Can you work these out from the model? Positions are in its coordinate system, mm. Face numbers are marked on the shaded views. A direction names the side the tool comes from. Round coordinates to 2 decimals unless told otherwise and drop trailing zeros. Write each loop counter-clockwise with the first axis right and the second up, starting at its lowest first coordinate (ties: lowest second). Pieces come first, ordered by that corner, then holes.
Q1. If we section it at B-B (z = 4): Please give me the cut outline in (x, y), plus the area to 3 significant figures.
Q2. We'd pull the mould along Y, two halves only. Please class the marked faces 1, 2, 3 and 4: +Y half, -Y half, draft (parallel to the pull), parting line (faces both ways), or undercut.
Q3. For the marked faces 5, 6 and 7, which set-ups out of +Z, -Z, +X, -X, +Y, -Y let a thin tool reach every point of the face, with its end or its side?
Q4. If we section it at D-D (y = 0.5): Please give me the cut outline in (x, z).
Q5. If we section it at A-A (x = -9.5): Please give me the cut outline in (y, z).
Q6. Please list where these lines run through material, in increasing order: line 1 along Y through (x, z) = (1.75, 26.75); line 2 along Z through (x, y) = (-7.5, -0.25); line 3 along Z through (x, y) = (0, 4.3).
Q7. If we section it at C-C (z = 9.5): Please give me the cut outline in (x, y).
Q8. I'm going to push flat-ended pins straight in: pin 1 Ø2.5 at (x, y) = (0, 0) entering from -Z; pin 2 Ø1.8 at (y, z) = (-0.5, 5) entering from -X; pin 3 Ø4 at (x, y) = (0, -1.5) entering from +Z. Where does each tip first touch, or does it pass through?
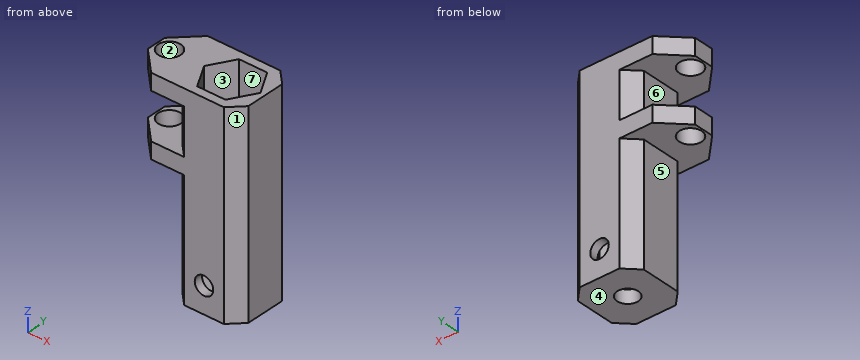
from build123d import *

# Parameters (mm, degrees)
ESQUISSE1_W             = 10
ESQUISSE1_H             = 10
BOSS_EXTRU_1_DEPTH      = 30
ENL_V_MAT_EXTRU_1_DEPTH = 28
ESQUISSE3_R             = 1.6
ENL_V_MAT_EXTRU_2_DEPTH = 31.822070015
ESQUISSE4_W             = 2.5
ESQUISSE4_H             = 10
BOSS_EXTRU_2_DEPTH      = 6.5
CHANFREIN2_SIZE         = 3.5
ESQUISSE5_R             = 1.7
ENL_V_MAT_EXTRU_3_DEPTH = 22.937410968
CHANFREIN3_SIZE         = 2
ESQUISSE9_R             = 1.4
ENL_V_MAT_EXTRU_4_DEPTH = 10


with BuildPart() as part:
    # Esquisse1 → Boss.-Extru.1 (new body)
    with BuildSketch(Plane.XY):
        Rectangle(ESQUISSE1_W, ESQUISSE1_H)
    extrude(amount=BOSS_EXTRU_1_DEPTH)

    # Esquisse2 → Enlèv. mat.-Extru.1 (cut)
    with BuildSketch(Plane.XY.offset(30)):
        Polygon((-4.272391992, 0), (-2.136195996, -3.7), (2.136195996, -3.7), (4.272391992, 0), (2.136195996, 3.7), (-2.136195996, 3.7), align=None)
    extrude(amount=-ENL_V_MAT_EXTRU_1_DEPTH, mode=Mode.SUBTRACT)

    # Esquisse3 → Enlèv. mat.-Extru.2 (cut, through all)
    with BuildSketch(Plane(origin=(0, 0, 0), x_dir=(-1, 0, 0), z_dir=(0, 0, -1))):
        Circle(ESQUISSE3_R)
    extrude(amount=-ENL_V_MAT_EXTRU_2_DEPTH, mode=Mode.SUBTRACT)

    # Esquisse4 → Boss.-Extru.2 (add)
    with BuildSketch(Plane.ZY.offset(5)):
        with Locations((28.75, 0)):
            Rectangle(ESQUISSE4_W, ESQUISSE4_H)
        with Locations((19.25, 0)):
            Rectangle(ESQUISSE4_W, ESQUISSE4_H)
    extrude(amount=BOSS_EXTRU_2_DEPTH)

    # Chanfrein2
    chanfrein2_edges = [part.edges().sort_by_distance(p)[0] for p in [
        (-11.5, -5, 28.75),
        (-11.5, 5, 28.75),
        (-11.5, -5, 19.25),
        (-11.5, 5, 19.25),
    ]]
    chamfer(chanfrein2_edges, length=CHANFREIN2_SIZE)

    # Esquisse5 → Enlèv. mat.-Extru.3 (cut, through all)
    with BuildSketch(Plane(origin=(0, 0, 18), x_dir=(-1, 0, 0), z_dir=(0, 0, -1))):
        with Locations(Location((9.5, 0, 0), (0, 0, 90))):
            Circle(ESQUISSE5_R)
    extrude(amount=-ENL_V_MAT_EXTRU_3_DEPTH, mode=Mode.SUBTRACT)

    # Chanfrein3
    chanfrein3_edges = [part.edges().sort_by_distance(p)[0] for p in [
        (-5, 5, 24),
        (-5, -5, 24),
        (5, -5, 15),
        (5, 5, 15),
        (-5, 5, 9),
        (-5, -5, 9),
    ]]
    chamfer(chanfrein3_edges, length=CHANFREIN3_SIZE)

    # Esquisse9 → Enlèv. mat.-Extru.4 (cut)
    with BuildSketch(Plane(origin=(0, 5, 0), x_dir=(1, 0, 0), z_dir=(0, 1, 0))):
        with Locations(Location((0, -4, 0), (0, 0, 180))):
            Circle(ESQUISSE9_R)
    extrude(amount=-ENL_V_MAT_EXTRU_4_DEPTH, mode=Mode.SUBTRACT)


solid = part.part
A:
1. outline: (-5, -3) - (-3, -5) - (-1.4, -5) - (-1.4, -3.7) - (-2.14, -3.7) - (-4.27, 0) - (-2.14, 3.7) - (-1.4, 3.7) - (-1.4, 5) - (-3, 5) - (-5, 3) - close; (1.4, -5) - (3, -5) - (5, -3) - (5, 3) - (3, 5) - (1.4, 5) - (1.4, 3.7) - (2.14, 3.7) - (4.27, 0) - (2.14, -3.7) - (1.4, -3.7) - close
1. area: 37.3 mm2
2. face 1: -Y half
2. face 2: undercut
2. face 3: undercut
2. face 4: draft
3. face 5: -Z, -X, +Y, -Y
3. face 6: -X, +Y, -Y
3. face 7: +Z
4. outline: (-11.5, 18) - (-11.12, 18) - (-11.12, 20.5) - (-11.5, 20.5) - close; (-11.5, 27.5) - (-11.12, 27.5) - (-11.12, 30) - (-11.5, 30) - close; (-7.88, 18) - (-5, 18) - (-5, 0) - (-1.52, 0) - (-1.52, 2) - (-3.98, 2) - (-3.98, 30) - (-7.88, 30) - (-7.88, 27.5) - (-5, 27.5) - (-5, 20.5) - (-7.88, 20.5) - close; (1.52, 0) - (5, 0) - (5, 30) - (3.98, 30) - (3.98, 2) - (1.52, 2) - close
5. outline: (-3.5, 18) - (-1.7, 18) - (-1.7, 20.5) - (-3.5, 20.5) - close; (-3.5, 27.5) - (-1.7, 27.5) - (-1.7, 30) - (-3.5, 30) - close; (1.7, 18) - (3.5, 18) - (3.5, 20.5) - (1.7, 20.5) - close; (1.7, 27.5) - (3.5, 27.5) - (3.5, 30) - (1.7, 30) - close
6. line 1: y = -5 to -3.7, 3.7 to 5
6. line 2: z = 18 to 20.5, 27.5 to 30
6. line 3: z = 0 to 2.6, 5.4 to 30
7. outline: (-5, -3) - (-3, -5) - (3, -5) - (5, -3) - (5, 3) - (3, 5) - (-3, 5) - (-5, 3) - close; hole (-4.27, 0) - (-2.14, -3.7) - (2.14, -3.7) - (4.27, 0) - (2.14, 3.7) - (-2.14, 3.7) - close
8. pin 1: passes through
8. pin 2: stops at x = -5
8. pin 3: stops at z = 2
